Can you work these out from the model? Positions are in its coordinate system, mm. Give positions to 0.01 mm unless a question says otherwise; leave off trailing zeros. Write each loop counter-clockwise with the first axis right and the second up, starting at its lowest first coordinate (ties: lowest second). Pieces come first, ordered by that corner, then holes.
```python
from build123d import *

# Parameters (mm, degrees)
SKETCH1_W           = 17
SKETCH1_H           = 23
BOSS_EXTRUDE1_DEPTH = 3
SKETCH2_R           = 1.5
SKETCH2_R_2         = 0.5
CUT_EXTRUDE1_DEPTH  = 4
SKETCH3_R           = 1.75
CUT_EXTRUDE2_DEPTH  = 4


with BuildPart() as part:
    # Sketch1 → Boss-Extrude1 (new body)
    with BuildSketch(Plane(origin=(0, 0, 0), x_dir=(1, 0, 0), z_dir=(0, 1, 0))):
        Rectangle(SKETCH1_W, SKETCH1_H)
    extrude(amount=BOSS_EXTRUDE1_DEPTH)

    # Sketch2 → Cut-Extrude1 (cut, through all)
    with BuildSketch(Plane(origin=(0, 3, 0), x_dir=(1, 0, 0), z_dir=(0, 1, 0))):
        with Locations((0, 9)):
            Circle(SKETCH2_R)
        with Locations((0, 4.4)):
            Circle(SKETCH2_R_2)
        with Locations((0, -4.4)):
            Circle(SKETCH2_R_2)
        with Locations((0, -9)):
            Circle(SKETCH2_R)
    extrude(amount=-CUT_EXTRUDE1_DEPTH, mode=Mode.SUBTRACT)

    # Sketch3 → Cut-Extrude2 (cut, through all)
    with BuildSketch(Plane(origin=(0, 3, 0), x_dir=(1, 0, 0), z_dir=(0, 1, 0))):
        Circle(SKETCH3_R)
    extrude(amount=-CUT_EXTRUDE2_DEPTH, mode=Mode.SUBTRACT)


solid = part.part
```
1) If we mould it in two halves opening along Z, with no side actions, what happens to faces 1 (the face through (0, 1, -11.5)), 2 (the face through (0, 1, 11.5)), 3 (the face through (-0.325, 1.521, -7.536)), 4 (the face through (-2, 0, 0))? For each: +Z half, -Z half, draft (parallel to the pull), parting line (faces both ways), or undercut.
Values follow:
face 1: -Z half
face 2: +Z half
face 3: undercut
face 4: draft
2) Suppose I cut it at D-D on z = 9. Write out the boundary of the cut face in (x, y).
Values follow:
outline: (-8.5, 0) - (-1.5, 0) - (-1.5, 3) - (-8.5, 3) - close; (1.5, 0) - (8.5, 0) - (8.5, 3) - (1.5, 3) - close
3) Suppose I cut it at B-B on x = 0. Write out the boundary of the cut face in (y, z), plus the area to 3 significant figures.
Values follow:
outline: (0, -11.5) - (3, -11.5) - (3, -10.5) - (0, -10.5) - close; (0, -7.5) - (3, -7.5) - (3, -4.9) - (0, -4.9) - close; (0, -3.9) - (3, -3.9) - (3, -1.75) - (0, -1.75) - close; (0, 1.75) - (3, 1.75) - (3, 3.9) - (0, 3.9) - close; (0, 4.9) - (3, 4.9) - (3, 7.5) - (0, 7.5) - close; (0, 10.5) - (3, 10.5) - (3, 11.5) - (0, 11.5) - close
area: 34.5 mm2
4) Please list where these lines run through material, in increasing order: L1, parallel to Z at x = 0, y = 1.95; L2, parallel to X at y = 1.65, z = -4.4; L3, parallel to X at y = 1.6, z = -9.
Values follow:
L1: z = -11.5 to -10.5, -7.5 to -4.9, -3.9 to -1.75, 1.75 to 3.9, 4.9 to 7.5, 10.5 to 11.5
L2: x = -8.5 to -0.5, 0.5 to 8.5
L3: x = -8.5 to -1.5, 1.5 to 8.5
5) Suppose I cut it at A-A on z = -4.4. Write out the boundary of the cut face in (x, y), plus the area to 3 significant figures.
Values follow:
outline: (-8.5, 0) - (-0.5, 0) - (-0.5, 3) - (-8.5, 3) - close; (0.5, 0) - (8.5, 0) - (8.5, 3) - (0.5, 3) - close
area: 48.0 mm2
6) Suppose I cut it at C-C on y = 1.95. Write out the boundary of the cut face in (x, z).
Values follow:
outline: (-8.5, -11.5) - (8.5, -11.5) - (8.5, 11.5) - (-8.5, 11.5) - close; hole circle Ø3.5 at (0, 0); hole circle Ø3 at (0, -9); hole circle Ø3 at (0, 9); hole circle Ø1 at (0, -4.4); hole circle Ø1 at (0, 4.4)
